Here's how the part is built. I have some questions about the finished solid (model axes, mm). A direction names the side the tool comes from. Coordinates: 2 decimals unless noted, no trailing zeros. Write each loop counter-clockwise with the first axis right and the second up, starting at its lowest first coordinate (ties: lowest second). Pieces come first, ordered by that corner, then holes. Notation, with made-up numbers: (86.25, 63.5) -> (95.25, 63.5) arc R20 ccw to (95.25, 90.5) -> close; hole circle Ø6 at (12, 24.25). An arc over 180 degrees is marked (long way). Put each result on its own line as item: value. Start each with the question number.
Item 1: For pin 1 (3 mm diameter, centred on x = 4, y = 0, fed in from -Z), with a flat end and sliding along its axis, tell me the tip position at first contact or that it passes through.
Item 2: On a 3-axis mill with a long thin cutter (end or side, diameter ignored), from which of +Z, -Z, +X, -X, +Y, -Y can I reach the whole of each face in a straight line? I mean faces 1 (the face through (3.015, 4.715, 2.299)), 2 (the face through (3.161, -4.715, 2.299)), 3 (the face through (0, 0, 3)). Say none if no direction works.
Item 3: I need wall thicknesses on line 1 (Z direction, x = 11, y = 3); line 2 (Y direction, x = -6.75, z = 1.05); line 3 (X direction, y = -2.5, z = 0.3). Which ranges of each line are inside material? Lowest first, please. Write a range as [from, to].
Item 4: I want a section at A-A, the plane x = 7.75. List the corners of the cut face in (y, z) for me.
from build123d import *

# Parameters (mm, degrees)
BOSS_EXTRUDE7_DEPTH  = 2.5
BOSS_EXTRUDE8_DEPTH  = 4.4
FILLET1_R            = 0.2
FILLET2_R            = 0.2
BOSS_EXTRUDE9_DEPTH  = 4.4
BOSS_EXTRUDE10_DEPTH = 2.6
FILLET3_R            = 1


with BuildPart() as part:
    # Sketch1 → Boss-Extrude7 (new body)
    with BuildSketch(Plane.XY):
        with BuildLine():
            ThreePointArc((-8.105508314, 3.661777672), (-4.68058624, 3.096358858), (-3.111398084, 0))
            Line((-3.111398084, 0), (0, 0))
            ThreePointArc((0, 0), (-0.552546694, 2.715894232), (-2.12233973, 5))
            Line((-2.12233973, 5), (-4.700896107, 5))
            ThreePointArc((-4.700896107, 5), (-6.529982168, 4.65343359), (-8.105508314, 3.661777672))
        make_face()
    extrude(amount=BOSS_EXTRUDE7_DEPTH)

    # Sketch1_7 → Boss-Extrude8 (add)
    with BuildSketch(Plane.XY):
        with BuildLine():
            ThreePointArc((-9.512562774, 1.359361574), (-6.250479564, 2.814145815), (-4.050896107, 0))
            Line((-4.050896107, 0), (-3.111398084, 0))
            ThreePointArc((-3.111398084, 0), (-4.68058624, 3.096358858), (-8.105508314, 3.661777672))
            ThreePointArc((-8.105508314, 3.661777672), (-8.967286807, 2.607280268), (-9.512562774, 1.359361574))
        make_face()
        with BuildLine():
            Line((-3.111398084, 0), (-4.050896107, 0))
            ThreePointArc((-4.050896107, 0), (-6.250479564, -2.814145815), (-9.512562774, -1.359361574))
            ThreePointArc((-9.512562774, -1.359361574), (-8.967286807, -2.607280268), (-8.105508314, -3.661777672))
            ThreePointArc((-8.105508314, -3.661777672), (-4.68058624, -3.096358858), (-3.111398084, 0))
        make_face()
    extrude(amount=BOSS_EXTRUDE8_DEPTH)

    # Fillet1
    fillet1_edges = [part.edges().sort_by_distance(p)[0] for p in [
        (-9.512562774, -1.359361574, 2.2),
    ]]
    fillet(fillet1_edges, radius=FILLET1_R)

    # Fillet2
    fillet2_edges = [part.edges().sort_by_distance(p)[0] for p in [
        (-9.512562774, 1.359361574, 2.2),
    ]]
    fillet(fillet2_edges, radius=FILLET2_R)

    # Sketch1_8 → Boss-Extrude9 (add)
    with BuildSketch(Plane.XY):
        with BuildLine():
            ThreePointArc((-8.105508314, 3.661777672), (-4.68058624, 3.096358858), (-3.111398084, 0))
            Line((-3.111398084, 0), (0, 0))
            ThreePointArc((0, 0), (-0.552546694, 2.715894232), (-2.12233973, 5))
            Line((-2.12233973, 5), (-4.700896107, 5))
            ThreePointArc((-4.700896107, 5), (-6.529982168, 4.65343359), (-8.105508314, 3.661777672))
        make_face()
        with BuildLine():
            Line((0, 0), (-3.111398084, 0))
            ThreePointArc((-3.111398084, 0), (-4.68058624, -3.096358858), (-8.105508314, -3.661777672))
            ThreePointArc((-8.105508314, -3.661777672), (-6.529982168, -4.65343359), (-4.700896107, -5))
            Line((-4.700896107, -5), (-2.12233973, -5))
            ThreePointArc((-2.12233973, -5), (-0.552546694, -2.715894232), (0, 0))
        make_face()
    extrude(amount=BOSS_EXTRUDE9_DEPTH)

    # Sketch1_12 → Boss-Extrude10 (add)
    with BuildSketch(Plane.XY):
        with BuildLine():
            Line((8.299103893, 5), (-2.12233973, 5))
            ThreePointArc((-2.12233973, 5), (-0.552546694, 2.715894232), (0, 0))
            ThreePointArc((0, 0), (-0.552546694, -2.715894232), (-2.12233973, -5))
            Line((-2.12233973, -5), (8.299103893, -5))
            ThreePointArc((8.299103893, -5), (13.299103893, 0), (8.299103893, 5))
        make_face()
    extrude(amount=BOSS_EXTRUDE10_DEPTH)

    # Fillet3
    fillet3_edges = [part.edges().sort_by_distance(p)[0] for p in [
        (3.088382082, 5, 2.6),
        (3.088382082, -5, 2.6),
        (13.299103893, 0, 2.6),
    ]]
    fillet(fillet3_edges, radius=FILLET3_R)


solid = part.part
Calculated:
1. pin 1: stops at z = 0
2. face 1: +Z, +X, +Y
2. face 2: +Z, +X, -Y
2. face 3: +Z, +X
3. line 1: z = [0, 2.6]
3. line 2: y = [-4.56, -2.89], [2.89, 4.56]
3. line 3: x = [-9.01, -8.42], [-5.48, 12.63]
4. outline: (-5, 0) -> (5, 0) -> (5, 1.6) arc R1 ccw to (4, 2.6) -> (-4, 2.6) arc R1 ccw to (-5, 1.6) -> close
